Answer from the drawing. Dimensions are ordinates in mm from the lowest x, y and z of the part. A direction names the side the tool comes from. Give positions to 0.01 mm unless a question says otherwise; leave off trailing zeros. Order: outer loops, then holes, each group sorted by start corner. A loop starts at its lowest first (then second) coordinate and runs counter-clockwise, first axis right, second up. Notation, with made-up numbers: (36, -14) -> (54, -14) arc R31 ccw to (54, 13) -> close; hole circle Ø6 at (-12, 85). An arc over 180 degrees is marked (long way). Answer as CSV lines item,"result". Start each with the question number.
1) Find section B-B (x = 34). Determine the outline of the cut face in (y, z) (1 decimal), and give its area (3 significant figures).
2) Straight lines are drawn through the part: L1, parallel to X at y = 26.5, z = 11 (1 decimal); L2, parallel to Y at x = 56, z = 13 (1 decimal); L3, parallel to X at y = 83, z = 33.5 (1 decimal). For each, find the intervals that lie inside material, in ascending order. Write a range as from..to.
3) Find section C-C (y = 72.5). Determine the outline of the cut face in (x, z) (1 decimal).
4) Flat-ended cylindrical pins translate along their axes: pin 1 Ø0.9 at (y, z) = (90.5, 11.5) entering from +X (1 decimal); pin 2 Ø6 at (y, z) = (83, 13.5) entering from -X; pin 3 Ø4 at (y, z) = (79, 28) entering from -X; pin 4 Ø1.5 at (x, y) = (37.5, 90.5) entering from -Z. Find the tip coordinate at first contact, or state that the pin passes through.
5) The mould has two halves that part along X. Classify the marked faces 1, 2 and 3: +X half, -X half, draft (parallel to the pull), parting line (faces both ways), or undercut.
6) For the marked faces 4 and 5, determine the directions among +Z, -Z, +X, -X, +Y, -Y from which every point of the face is accessible in a straight line to the end or side of a thin tool.
7) Find section D-D (z = 10). Determine the outline of the cut face in (x, y) (1 decimal), and give its area (3 significant figures).
8) Find section A-A (x = 121). Determine the outline of the cut face in (y, z) (1 decimal), and give its area (3 significant figures).
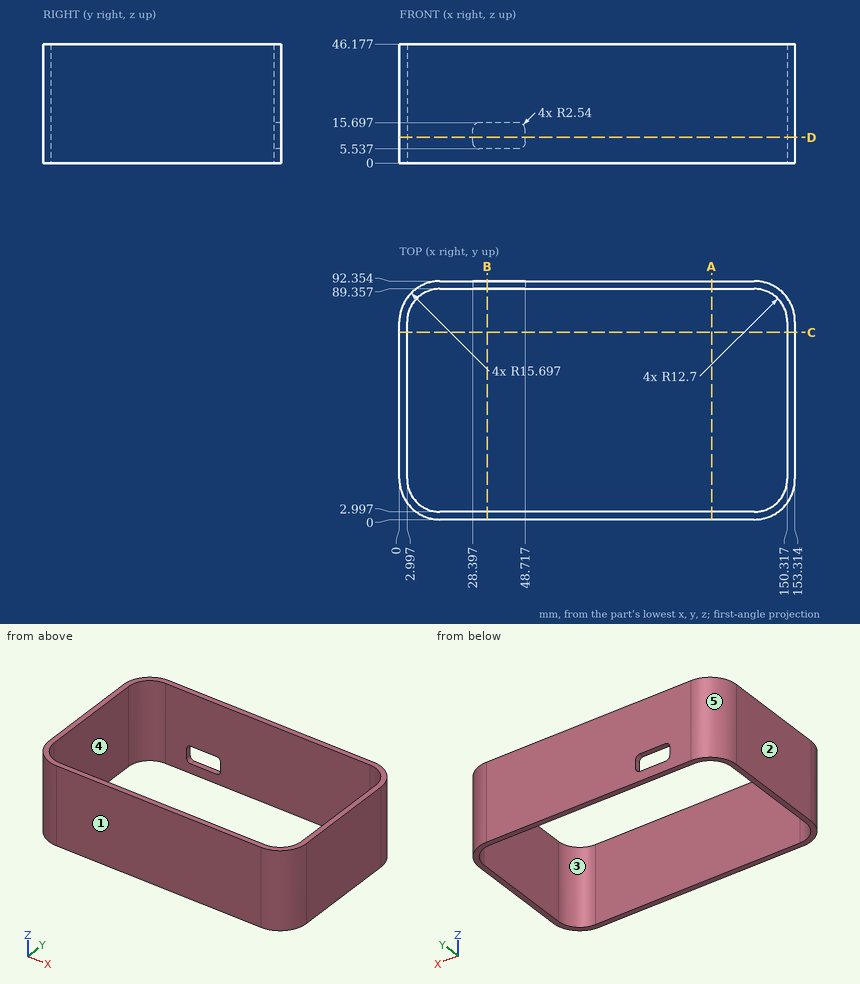
Findings below:
1,outline,"(0, 0) -> (3, 0) -> (3, 46.2) -> (0, 46.2) -> close; (89.4, 0) -> (92.4, 0) -> (92.4, 5.5) -> (89.4, 5.5) -> close; (89.4, 15.7) -> (92.4, 15.7) -> (92.4, 46.2) -> (89.4, 46.2) -> close"
1,area,"246 mm²"
2,L1,"0..3, 150.3..153.3"
2,L2,"0..3, 89.4..92.4"
2,L3,"1.3..4.7, 148.6..152"
3,outline,"(0, 0) -> (3, 0) -> (3, 46.2) -> (0, 46.2) -> close; (150.3, 0) -> (153.3, 0) -> (153.3, 46.2) -> (150.3, 46.2) -> close"
4,pin 1,"x = 145.8"
4,pin 2,"x = 0.36"
4,pin 3,"x = 0"
4,pin 4,"z = 0"
5,face 1,"draft"
5,face 2,"-X half"
5,face 3,"undercut"
6,face 4,"+Z, -Z"
6,face 5,"+Z, -Z, -X, +Y"
7,outline,"(0, 15.7) arc R15.7 ccw to (15.7, 0) -> (137.6, 0) arc R15.7 ccw to (153.3, 15.7) -> (153.3, 76.7) arc R15.7 ccw to (137.6, 92.4) -> (48.7, 92.4) -> (48.7, 89.4) -> (137.6, 89.4) arc R12.7 cw to (150.3, 76.7) -> (150.3, 15.7) arc R12.7 cw to (137.6, 3) -> (15.7, 3) arc R12.7 cw to (3, 15.7) -> (3, 76.7) arc R12.7 cw to (15.7, 89.4) -> (28.4, 89.4) -> (28.4, 92.4) -> (15.7, 92.4) arc R15.7 ccw to (0, 76.7) -> close"
7,area,"1,300 mm²"
8,outline,"(0, 0) -> (3, 0) -> (3, 46.2) -> (0, 46.2) -> close; (89.4, 0) -> (92.4, 0) -> (92.4, 46.2) -> (89.4, 46.2) -> close"
8,area,"277 mm²"
